Check sheet for the drawn part. Datum: minimum x, y, z corner. Units: mm. A direction names the side the tool comes from. Round coordinates to 2 decimals unless told otherwise and drop trailing zeros. Order: outer loops, then holes, each group sorted by start corner. A loop starts at its lowest first (then second) coordinate and runs counter-clockwise, first axis right, second up. Notation, with made-up numbers: (-39.5, -15.5) - (-6.5, -15.5) arc R17 ccw to (-6.5, 8.5) - close; hole circle Ø5 at (33, 86.25). An arc over 180 degrees is marked (long way). Write each question's results on one line, items separated by ' | '.
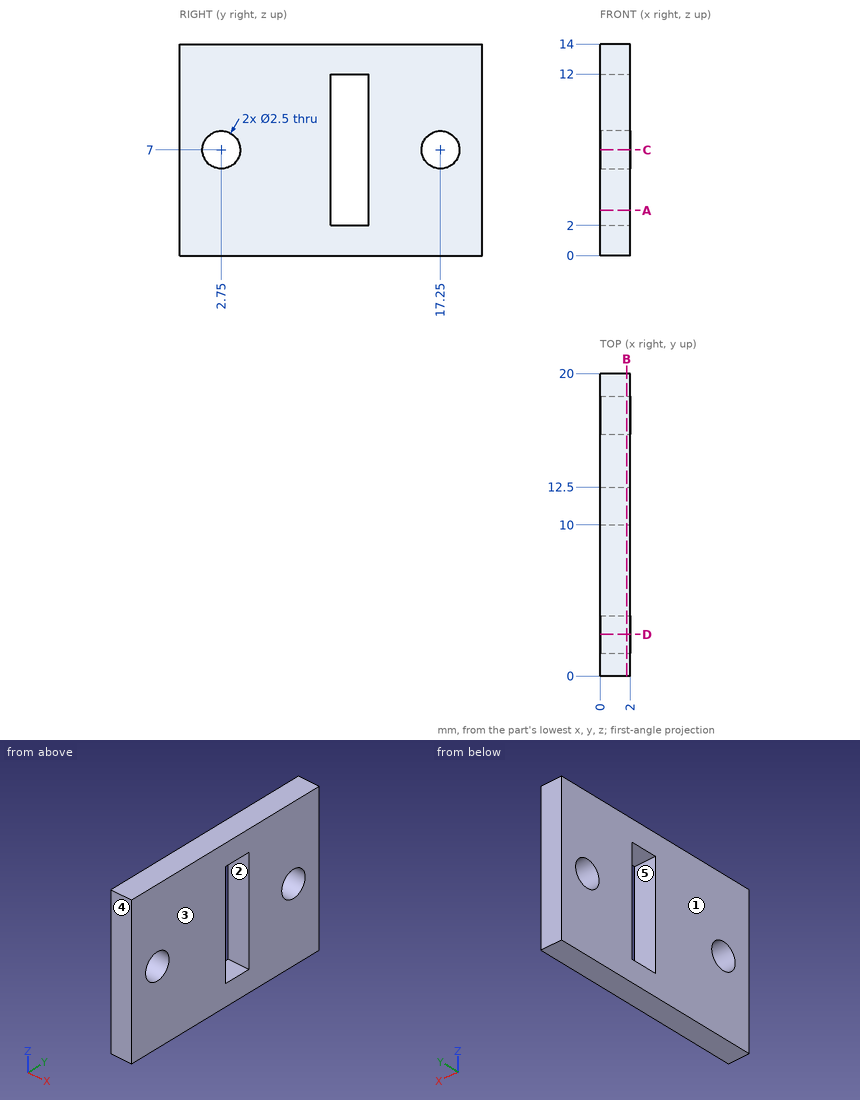
(1) Draft check along Y on the marked faces 3, 4 and 5. Enter one of: released by +Y, released by -Y, zero draft, split by the parting line, or undercut.
Answers follow:
face 3: zero draft | face 4: released by -Y | face 5: undercut
(2) Section check A-A (z = 3). Record the cut outline in (x, y), then the cut area to 3 significant figures.
Answers follow:
outline: (0, 0) - (2, 0) - (2, 10) - (0, 10) - close; (0, 12.5) - (2, 12.5) - (2, 20) - (0, 20) - close | area: 35.0 mm²
(3) Material ranges on line 1 (Y direction, x = 0.9, z = 7); line 2 (Y direction, x = 1.9, z = 10.25); line 3 (Y direction, x = 1.75, z = 8), recorded low to high.
Answers follow:
line 1: 0 to 1.5, 4 to 10, 12.5 to 16, 18.5 to 20 | line 2: 0 to 10, 12.5 to 20 | line 3: 0 to 2, 3.5 to 10, 12.5 to 16.5, 18 to 20
(4) Section check C-C (z = 7). Record the cut outline in (x, y).
Answers follow:
outline: (0, 0) - (2, 0) - (2, 1.5) - (0, 1.5) - close; (0, 4) - (2, 4) - (2, 10) - (0, 10) - close; (0, 12.5) - (2, 12.5) - (2, 16) - (0, 16) - close; (0, 18.5) - (2, 18.5) - (2, 20) - (0, 20) - close
(5) Section check B-B (x = 1.75). Record the cut outline in (y, z), then the cut area to 3 significant figures.
Answers follow:
outline: (0, 0) - (20, 0) - (20, 14) - (0, 14) - close; hole circle Ø2.5 at (2.75, 7); hole (10, 2) - (12.5, 2) - (12.5, 12) - (10, 12) - close; hole circle Ø2.5 at (17.25, 7) | area: 245 mm²
(6) Section check D-D (y = 2.75). Record the cut outline in (x, z), then the cut area to 3 significant figures.
Answers follow:
outline: (0, 0) - (2, 0) - (2, 5.75) - (0, 5.75) - close; (0, 8.25) - (2, 8.25) - (2, 14) - (0, 14) - close | area: 23.0 mm²
(7) Access from +Z, -Z, +X, -X, +Y, -Y to the whole of each face (thin tool, end or side, straight path). Record for the marked faces 1 and 2.
Answers follow:
face 1: +Z, -Z, -X, +Y, -Y | face 2: +X, -X
(8) Depth check by flat-ended pin: pin 1 Ø3 at (y, z) = (17.25, 7) entering from +X. Enter the tip coordinate at first touch or a pass-through.
Answers follow:
pin 1: x = 2
